Geometry: final body of the model. Coordinates: model frame, mm. Give positions to 0.01 mm unless a question says otherwise; leave off trailing zeros. Write each loop counter-clockwise with the first axis right and the second up, starting at its lowest first coordinate (ties: lowest second). Pieces come first, ordered by that corner, then holes.
Q1. Cut plane A-A on x = 0. Return the cut outline in (y, z) (3 decimals), plus the area to 3 significant figures.
Q2. Cut plane B-B on x = 101.6. Return the cut outline in (y, z).
Q3. Line query: L1, parallel to Y at x = 0, z = 4 (3 decimals); L2, parallel to Z at x = -2.5, y = 6; L3, parallel to Y at x = 101.6, z = 2. Output: solid intervals per line, ascending.
Q4. Pin query (flat end, axial travel): pin 1 (1.9 mm diameter, centred on x = -13, z = 9, fed in from -Y) (3 decimals); pin 2 (7.5 mm diameter, centred on x = -25.4, y = 0, fed in from +Z); pin 3 (1.4 mm diameter, centred on x = 17, z = 8.5, fed in from +Y) (3 decimals); pin 4 (5 mm diameter, centred on x = 101.6, y = -20.95, fed in from +Z). Return the tip coordinate at first contact, or that it passes through.
Q5. Cut plane C-C on x = 69.5. Return the cut outline in (y, z), plus the area to 3 significant figures.
```python
from build123d import *

# Parameters (mm, degrees)
SKETCH1_R               = 3.175
SKETCH1_R_2             = 4
BOSS_EXTRUDE1_DEPTH     = 6.35
CUT_EXTRUDE2_REACH      = 155.866
CUT_EXTRUDE2_END_RADIUS = 4
SKETCH3_R               = 1.1303
FILLET4_R               = 10
SKETCH4_W               = 6.35
SKETCH4_H               = 6.35
SKETCH4_W_2             = 19.05
BOSS_EXTRUDE2_DEPTH     = 4.7625
FILLET3_R               = 2


with BuildPart() as part:
    # Sketch1 → Boss-Extrude1 (new body)
    with BuildSketch(Plane.XY):
        Polygon((-38.1, -12.7), (-38.1, 12.7), (15.701735639, 12.7), (114.28491418, -10.930870684), (108.364133554, -35.631161305), (12.7, -12.7), align=None)
        with Locations((-25.4, 0)):
            Circle(SKETCH1_R, mode=Mode.SUBTRACT)
        Circle(SKETCH1_R, mode=Mode.SUBTRACT)
        with Locations((101.6, -20.95)):
            Circle(SKETCH1_R_2, mode=Mode.SUBTRACT)
    extrude(amount=BOSS_EXTRUDE1_DEPTH)

    # Cut-Extrude2: up to this cylinder (the profile starts outside it)
    cut_extrude2_end = Plane(origin=(101.6, -20.95, 3.175), z_dir=(0, 0, -1)) * Cylinder(CUT_EXTRUDE2_END_RADIUS, 320.732, mode=Mode.PRIVATE)
    # Sketch3 → Cut-Extrude2 (cut, up to the surface)
    with BuildSketch(Plane(origin=(110.552900462, -26.500071647, 0), x_dir=(0, 0, -1), z_dir=(0.9724523866696595, -0.23310159943784806, 0)), mode=Mode.PRIVATE) as cut_extrude2_sk1:
        with Locations(Location((-3.175, 3.310245002, 0), (0, 0, 90))):
            Circle(SKETCH3_R)
    cut_extrude2_tool1 = extrude(cut_extrude2_sk1.sketch, amount=-CUT_EXTRUDE2_REACH, mode=Mode.PRIVATE) - cut_extrude2_end
    add(cut_extrude2_tool1.solids().sort_by_distance((111.324524, -23.281016, 3.175))[0], mode=Mode.SUBTRACT)

    # Fillet4
    fillet4_edges = [part.edges().sort_by_distance(p)[0] for p in [
        (108.364133554, -35.631161305, 3.175),
        (114.28491418, -10.930870684, 3.175),
    ]]
    fillet(fillet4_edges, radius=FILLET4_R)

    # Sketch4 → Boss-Extrude2 (add)
    with BuildSketch(Plane.XY.offset(6.35)):
        with Locations((-12.7, 0)):
            Rectangle(SKETCH4_W, SKETCH4_H)
        with Locations((19.05, 0)):
            Rectangle(SKETCH4_W_2, SKETCH4_H)
    extrude(amount=BOSS_EXTRUDE2_DEPTH)

    # Fillet3
    fillet3_edges = [part.edges().sort_by_distance(p)[0] for p in [
        (12.7, -12.7, 3.175),
        (-38.1, -12.7, 3.175),
        (-38.1, 12.7, 3.175),
        (15.701735639, 12.7, 3.175),
        (-15.875, -3.175, 8.73125),
        (-9.525, -3.175, 8.73125),
        (-9.525, 3.175, 8.73125),
        (-15.875, 3.175, 8.73125),
        (9.525, -3.175, 8.73125),
        (28.575, -3.175, 8.73125),
        (28.575, 3.175, 8.73125),
        (9.525, 3.175, 8.73125),
    ]]
    fillet(fillet3_edges, radius=FILLET3_R)


solid = part.part
```
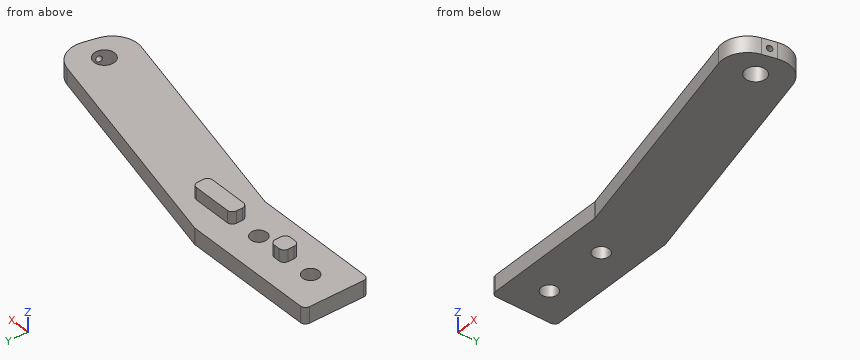
Data:
1. outline: (-12.7, 0) - (-3.175, 0) - (-3.175, 6.35) - (-12.7, 6.35) - close; (3.175, 0) - (12.7, 0) - (12.7, 6.35) - (3.175, 6.35) - close
1. area: 121 mm2
2. outline: (-33.56, 0) - (-24.95, 0) - (-24.95, 6.35) - (-33.56, 6.35) - close; (-16.95, 0) - (-7.89, 0) - (-7.89, 6.35) - (-16.95, 6.35) - close
3. L1: y = -12.7 to -3.175, 3.175 to 12.7
3. L2: z = 0 to 6.35
3. L3: y = -33.56 to -24.95, -16.95 to -7.89
4. pin 1: stops at y = -3.175
4. pin 2: stops at z = 6.35
4. pin 3: stops at y = 3.175
4. pin 4: passes through
5. outline: (-26.32, 0) - (-0.2, 0) - (-0.2, 6.35) - (-26.32, 6.35) - close
5. area: 166 mm2
